Source: CAD feature listing. Evaluate the final solid. Frame: model axes, mm. Face numbers are marked on the shaded views. Round coordinates to 2 decimals unless told otherwise and drop trailing zeros. Order: outer loops, then holes, each group sorted by start corner. A loop starts at its lowest first (then second) coordinate and runs counter-clockwise, first axis right, second up. Notation, with made-up numbers: (-35.5, 19) -> (-8.5, 19) arc R10 ccw to (-8.5, 28) -> close; hole circle Ø1 at (65, -28). An arc over 180 degrees is marked (long way). Write item = value, one per line. Start each with the question number.
(1) Cut plane A-A on x = 0. Return the cut outline in (y, z).
(2) Ray query, line 1 (Y direction, x = 0, z = -3.5); line 2 (Z direction, x = 3.5, y = 2.5); line 3 (Y direction, x = 4, z = -2.95). Return the intervals inside material, ascending.
(3) Contact query for flat-ended pins moving along their axis: pin 1 Ø16 at (x, y) = (-2, 7) entering from -Z; pin 2 Ø2 at (x, y) = (-14.5, -21.5) entering from +Z. Output: stop coordinate, or through.
(4) Cut plane C-C on z = -4.25. Return the cut outline in (x, y).
(5) Draft query along Y for the marked faces 1, 2, 3 and 4. Return one class per face: released by +Y, released by -Y, zero draft, split by the parting line, or undercut.
from build123d import *


with BuildPart() as part:
    # Sketch2 → Revolve1 (revolve)
    with BuildSketch(Plane(origin=(0, 0, 0), x_dir=(1, 0, 0), z_dir=(0, 1, 0)), mode=Mode.PRIVATE) as revolve1_sk:
        with BuildLine():
            Line((0, 0), (25.1, 0))
            ThreePointArc((25.1, 0), (26.443502884, 0.556497116), (27, 1.9))
            Line((27, 1.9), (27, 2))
            Line((27, 2), (25, 2))
            Line((25, 2), (25, 5))
            Line((25, 5), (23, 5))
            Line((23, 5), (23, 2))
            Line((23, 2), (0, 2))
            Line((0, 2), (0, 0))
        make_face()
    revolve(revolve1_sk.sketch.rotate(Axis((0, 0, -2), (0, 0, 1)), 180), axis=Axis((0, 0, -2), (0, 0, 1)))


solid = part.part
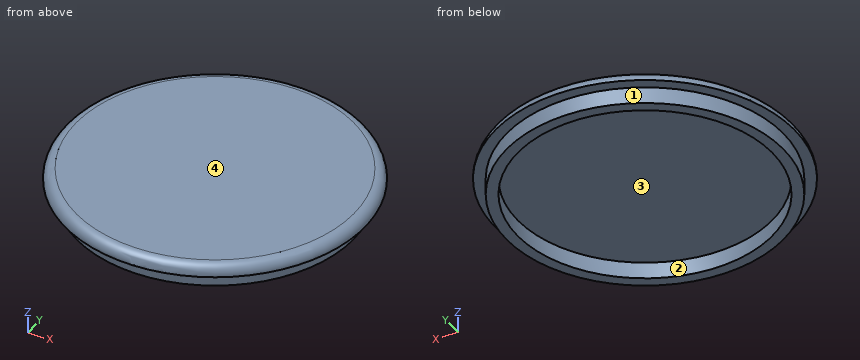
Evaluation:
q1.outline = (-27, -2) -> (-25, -2) -> (-25, -5) -> (-23, -5) -> (-23, -2) -> (23, -2) -> (23, -5) -> (25, -5) -> (25, -2) -> (27, -2) -> (27, -1.9) arc R1.9 ccw to (25.1, 0) -> (-25.1, 0) arc R1.9 ccw to (-27, -1.9) -> close
q2.line_1 = -25 to -23, 23 to 25
q2.line_2 = -2 to 0
q2.line_3 = -24.68 to -22.65, 22.65 to 24.68
q3.pin_1 = -2
q3.pin_2 = 0
q4.outline = circle Ø50 at (0, 0); hole circle Ø46 at (0, 0)
q5.face_1 = split by the parting line
q5.face_2 = undercut
q5.face_3 = undercut
q5.face_4 = zero draft
